Could you check a few things on this model? Use its own coordinates, in mm. Face numbers are marked on the shaded views. Round coordinates to 2 decimals unless told otherwise and drop trailing zeros. Order: outer loops, then holes, each group sorted by start corner. A loop starts at its lowest first (then second) coordinate and runs counter-clockwise, first axis right, second up. Notation, with made-up numbers: (30, -35.5) -> (40, -35.5) arc R13 ccw to (40, -12.5) -> close; hole circle Ø7 at (18.25, 78). An arc over 180 degrees is marked (long way). One line per question, with ' | ' between items.
```python
from build123d import *

# Parameters (mm, degrees)
SKETCH1_W           = 35
SKETCH1_H           = 195
BOSS_EXTRUDE1_DEPTH = 15
BOSS_EXTRUDE2_DEPTH = 2.5
BOSS_EXTRUDE3_START = 2.5
SKETCH3_R           = 2.125
BOSS_EXTRUDE3_DEPTH = 2.5
SKETCH4_W           = 30
SKETCH4_H           = 25
CUT_EXTRUDE1_DEPTH  = 260.5
SKETCH5_W           = 10.625
SKETCH5_H           = 15
CUT_EXTRUDE2_DEPTH  = 65
BOSS_EXTRUDE4_DEPTH = 10.625


with BuildPart() as part:
    # Sketch1 → Boss-Extrude1 (new body)
    with BuildSketch(Plane(origin=(0, 0, 0), x_dir=(1, 0, 0), z_dir=(0, 1, 0))):
        Rectangle(SKETCH1_W, SKETCH1_H)
    extrude(amount=BOSS_EXTRUDE1_DEPTH)

    # Sketch2 → Boss-Extrude2 (add)
    with BuildSketch(Plane.ZY.offset(17.5)):
        with BuildLine():
            ThreePointArc((95.375, 10.875), (94.75260191, 12.37760191), (93.25, 13))
            ThreePointArc((93.25, 13), (91.125, 10.875), (93.25, 8.75))
            ThreePointArc((93.25, 8.75), (94.75260191, 9.37239809), (95.375, 10.875))
        make_face()
    extrude(amount=BOSS_EXTRUDE2_DEPTH)

    # Sketch3 → Boss-Extrude3 (add)
    with BuildSketch(Plane(origin=(17.5, 0, 0), x_dir=(0, 0, -1), z_dir=(1, 0, 0)).offset(BOSS_EXTRUDE3_START)):
        with Locations((-93.25, 10.875)):
            Circle(SKETCH3_R)
    extrude(amount=-BOSS_EXTRUDE3_DEPTH)

    # Sketch4 → Cut-Extrude1 (cut)
    with BuildSketch(Plane.XY.offset(97.5)):
        Rectangle(SKETCH4_W, SKETCH4_H)
    extrude(amount=-CUT_EXTRUDE1_DEPTH, mode=Mode.SUBTRACT)

    # Sketch5 → Cut-Extrude2 (cut)
    with BuildSketch(Plane.ZY.offset(17.5)):
        with Locations((-92.1875, 7.5)):
            Rectangle(SKETCH5_W, SKETCH5_H)
    extrude(amount=-CUT_EXTRUDE2_DEPTH, mode=Mode.SUBTRACT)

    # Sketch6 → Boss-Extrude4 (add)
    with BuildSketch(Plane.XY.offset(97.5)):
        Polygon((-17.5, 15), (17.5, 15), (17.5, 0), (15, 0), (15, 12.5), (-15, 12.5), (-15, 0), (-17.5, 0), align=None)
    extrude(amount=BOSS_EXTRUDE4_DEPTH)


solid = part.part
```
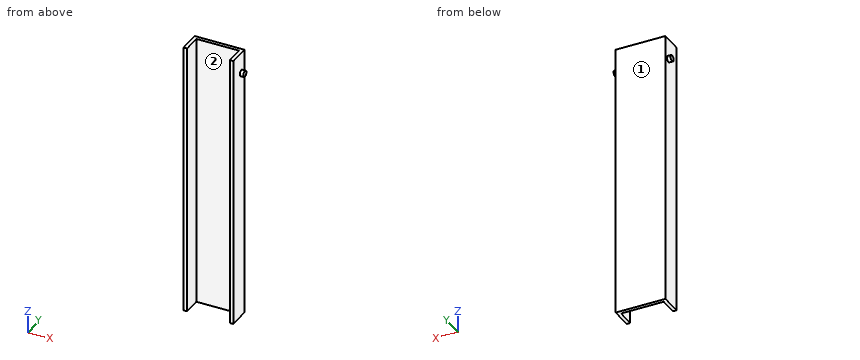
1. I'm going to push flat-ended pins straight in: pin 1 (5 mm diameter, centred on y = 4.5, z = 24, fed in from +X); pin 2 (5 mm diameter, centred on x = 0.5, z = 32, fed in from -Y). Where does each tip first touch, or does it pass through?
From the geometry:
pin 1: stops at x = 17.5 | pin 2: stops at y = 12.5
2. I want a section at C-C on x = -1. List the corners of the cut face in (y, z) for me (3 decimals), and give its area (4 significant figures).
From the geometry:
outline: (12.5, -86.875) -> (15, -86.875) -> (15, 108.125) -> (12.5, 108.125) -> close | area: 487.5 mm²
3. If we mould it in two halves opening along X, with no side actions, what happens to the marked faces 1 and 2? For each: pulls with the +X half, pulls with the -X half, needs draft (parallel to the pull), parting line crosses it, or undercut.
From the geometry:
face 1: needs draft | face 2: undercut
4. I want a section at A-A on y = 6.75. List the corners of the cut face in (x, z) for me (3 decimals).
From the geometry:
outline: (-17.5, -86.875) -> (-15, -86.875) -> (-15, 108.125) -> (-17.5, 108.125) -> close; (15, -86.875) -> (17.5, -86.875) -> (17.5, 108.125) -> (15, 108.125) -> close
5. I want a section at B-B on z = -25.5. List the corners of the cut face in (x, y) for me.
From the geometry:
outline: (-17.5, 0) -> (-15, 0) -> (-15, 12.5) -> (15, 12.5) -> (15, 0) -> (17.5, 0) -> (17.5, 15) -> (-17.5, 15) -> close
6. I need wall thicknesses on probe 1 along X at (y, z) = (11.5, -4); probe 2 along Y at (x, z) = (1, -72). Which ranges of each line are inside material? Lowest first, please.
From the geometry:
probe 1: x = -17.5 to -15, 15 to 17.5 | probe 2: y = 12.5 to 15
